from build123d import *

# Parameters (mm, degrees)
F1_DEPTH = 2


with BuildPart() as f1:
    # F0 (on Top) → F1 (new body)
    with BuildSketch(Plane.XY):
        with BuildLine():
            ThreePointArc((-38.974674, 23.580405), (-60.390278, -3.375836), (-64.951905, -37.5))
            ThreePointArc((-64.951905, -37.5), (-34.023862, -50.167524), (-0.874012, -45.913403))
            ThreePointArc((-0.874012, -45.913403), (-8.553201, -41.779684), (-15.62271, -36.672862))
            ThreePointArc((-15.62271, -36.672862), (-35.378352, -37.537867), (-54.126588, -31.25))
            ThreePointArc((-54.126588, -31.25), (-50.044813, -11.494391), (-39.013473, 5.395087))
            ThreePointArc((-39.013473, 5.395087), (-33.020374, 10.762858), (-26.297898, 15.183099))
            ThreePointArc((-26.297898, 15.183099), (-0.599358, 21.996682), (25.243749, 15.753792))
            ThreePointArc((25.243749, 15.753792), (25.772403, 15.471363), (26.297898, 15.183099))
            ThreePointArc((26.297898, 15.183099), (25.95057, 22.252358), (24.683909, 29.21588))
            Line((24.683909, 29.21588), (23.603483, 31.219872))
            ThreePointArc((23.603483, 31.219872), (-0.144813, 36.00849), (-23.990038, 31.728577))
            ThreePointArc((-23.990038, 31.728577), (-31.751976, 28.150327), (-38.974674, 23.580405))
        make_face()
        with BuildLine():
            ThreePointArc((39.555322, 21.859627), (26.997523, 53.803957), (0, 75))
            ThreePointArc((0, 75), (-26.171862, 54.356893), (-38.974674, 23.580405))
            ThreePointArc((-38.974674, 23.580405), (-31.751976, 28.150327), (-23.990038, 31.728577))
            ThreePointArc((-23.990038, 31.728577), (-14.863791, 49.350843), (0, 62.5))
            ThreePointArc((0, 62.5), (15.106633, 49.036989), (24.21408, 30.967195))
            ThreePointArc((24.21408, 30.967195), (24.456327, 30.093505), (24.683909, 29.21588))
            ThreePointArc((24.683909, 29.21588), (25.95057, 22.252358), (26.297898, 15.183099))
            ThreePointArc((26.297898, 15.183099), (26.283203, 14.526877), (26.260553, 13.870882))
            ThreePointArc((26.260553, 13.870882), (18.720926, -11.566447), (0, -30.366197))
            ThreePointArc((0, -30.366197), (7.342348, -34.040767), (15.155964, -36.562659))
            ThreePointArc((15.155964, -36.562659), (31.176915, -18), (39.242174, 5.155879))
            ThreePointArc((39.242174, 5.155879), (39.933917, 13.49772), (39.555322, 21.859627))
        make_face()
        with BuildLine():
            ThreePointArc((-0.874012, -45.913403), (31.493402, -51.705945), (62.657862, -41.218834))
            ThreePointArc((62.657862, -41.218834), (59.931979, -6.447298), (39.555322, 21.859627))
            ThreePointArc((39.555322, 21.859627), (39.933917, 13.49772), (39.242174, 5.155879))
            ThreePointArc((39.242174, 5.155879), (50.107668, -11.647461), (54.126588, -31.25))
            ThreePointArc((54.126588, -31.25), (35.140832, -37.570783), (15.155964, -36.562659))
            ThreePointArc((15.155964, -36.562659), (7.342348, -34.040767), (0, -30.366197))
            ThreePointArc((0, -30.366197), (-19.052559, -11), (-26.297898, 15.183099))
            ThreePointArc((-26.297898, 15.183099), (-33.020374, 10.762858), (-39.013473, 5.395087))
            ThreePointArc((-39.013473, 5.395087), (-31.274777, -17.838898), (-15.62271, -36.672862))
            ThreePointArc((-15.62271, -36.672862), (-8.553201, -41.779684), (-0.874012, -45.913403))
        make_face()
    extrude(amount=F1_DEPTH)


solid = f1.part
CAD build for the part. Positions are in the model's coordinates, mm. A direction names the side the tool comes from. Round coordinates to 2 decimals unless told otherwise and drop trailing zeros. Write each loop counter-clockwise with the first axis right and the second up, starting at its lowest first coordinate (ties: lowest second). Pieces come first, ordered by that corner, then holes. Notation, with made-up numbers: (69, 48.5) -> (103, 48.5) arc R26 ccw to (103, 63.5) -> close; hole circle Ø7 at (27, 69.5). An arc over 180 degrees is marked (long way). Answer as a JSON object with one key per item and string values.
(1) Band-saw the part on D-D, the plane y = -28.5. List the corners of the cut face in (x, z), then the cut area to 3 significant figures.
Reported:
{"outline": "(-65.55, 0) -> (-54.01, 0) -> (-54.01, 2) -> (-65.55, 2) -> close; (-23.89, 0) -> (-2.9, 0) -> (-2.9, 2) -> (-23.89, 2) -> close; (2.9, 0) -> (23.64, 0) -> (23.64, 2) -> (2.9, 2) -> close; (54.01, 0) -> (63.88, 0) -> (63.88, 2) -> (54.01, 2) -> close", "area": "126 mm^2"}
(2) Two-plate mould, pull along X, no slides. Class faces 3 (the face through (-16, -16, 0)), 4 (the face through (-25.886, 54.732, 0.986)), 5 (the face through (50, -11.39, 0.99)), 6 (the face through (0.196, 36.004, 0.986)): +X half, -X half, draft (parallel to the pull), parting line (faces both ways), or undercut.
Reported:
{"face 3": "draft", "face 4": "-X half", "face 5": "undercut", "face 6": "undercut"}
(3) Probe probe 1 along Y at (x, z) = (-18.5, 0.6) (3 decimals); probe 2 along Y at (x, z) = (-22, 0.5); probe 3 along X at (y, z) = (-8, 1.85). List the from-to ranges inside material, lowest first. Write a range as [from, to].
Reported:
{"probe 1": "y = [-50.349, -37.257], [-34.147, -11.935], [18.741, 33.555], [44.069, 62.843]", "probe 2": "y = [-50.63, -37.75], [-30.64, -5.09], [17.33, 32.45], [37.22, 59.33]", "probe 3": "x = [-62.15, -48.46], [-35.74, -20.66], [20.66, 35.87], [48.46, 60.48]"}
(4) Which spindle directions (+Z, -Z, +X, -X, +Y, -Y) get a long thin tool onto all of the face, cutting with end or side? Do faces 1 (the face through (-0.98, 21.99, 0.99)), 2 (the face through (-16, -16, 2)). Say none if no direction does.
Reported:
{"face 1": "+Z, -Z", "face 2": "+Z, +X, -X, +Y, -Y"}
(5) Band-saw the part on B-B, the plane x = -12. List the corners of the cut face in (y, z).
Reported:
{"outline": "(-49.32, 0) -> (-20.6, 0) -> (-20.6, 2) -> (-49.32, 2) -> close; (20.65, 0) -> (35.04, 0) -> (35.04, 2) -> (20.65, 2) -> close; (52.73, 0) -> (68.16, 0) -> (68.16, 2) -> (52.73, 2) -> close"}
(6) Band-saw the part on C-C, the plane z = 0.7. List the corners of the cut face in (x, y), then the cut area to 3 significant figures.
Reported:
{"outline": "(-64.95, -37.5) arc R65.45 ccw to (-0.87, -45.91) arc R66.23 ccw to (62.66, -41.22) arc R64.72 ccw to (39.56, 21.86) arc R65.45 ccw to (0, 75) arc R66.23 ccw to (-38.97, 23.58) arc R64.72 ccw to start; hole (-54.13, -31.25) arc R54.13 ccw to (-15.62, -36.67) arc R66.23 cw to (-39.01, 5.4) arc R54.13 ccw to start; hole (-26.3, 15.18) arc R54.13 ccw to (0, -30.37) arc R54.13 ccw to (26.26, 13.87) arc R54.14 ccw to (26.3, 15.18) arc R54.14 ccw to (25.24, 15.75) arc R54.13 ccw to start; hole (-23.99, 31.73) arc R64.72 cw to (23.6, 31.22) -> (24.68, 29.22) arc R54.14 ccw to (24.21, 30.97) arc R54.13 ccw to (0, 62.5) arc R54.13 ccw to start; hole (15.16, -36.56) arc R54.13 ccw to (54.13, -31.25) arc R54.13 ccw to (39.24, 5.16) arc R65.45 cw to start", "area": "6,890 mm^2"}
(7) Band-saw the part on A-A, the plane x = -47.5. List the corners of the cut face in (y, z), then the cut area to 3 significant figures.
Reported:
{"outline": "(-46.92, 0) -> (-34.37, 0) -> (-34.37, 2) -> (-46.92, 2) -> close; (-6.17, 0) -> (16.14, 0) -> (16.14, 2) -> (-6.17, 2) -> close", "area": "69.7 mm^2"}
